Can you work these out from the model? Positions are in its coordinate system, mm. Face numbers are marked on the shaded views. Give positions to 0.01 mm unless a question says otherwise; leave off trailing zeros. Loops run counter-clockwise (first coordinate to the right, second up) from the corner with the lowest first, then second, coordinate; pieces in that order, holes last. Notation, with made-up numbers: (87.25, 30.5) -> (118.25, 30.5) arc R28 ccw to (118.25, 62.5) -> close; hole circle Ø10 at (35, 21.25). An arc over 180 degrees is marked (long way). One line per question, with ' | ' between items.
from build123d import *

# Parameters (mm, degrees)
SKETCH1_W                     = 22.225
SKETCH1_H                     = 15.875
SKETCH1_R                     = 1.5875
BOSS_EXTRUDE1_DEPTH           = 1
SKETCH2_W                     = 3
SKETCH2_H                     = 4
BOSS_EXTRUDE2_DEPTH           = 1
SKETCH3_R                     = 1.27
BOSS_EXTRUDE3_DEPTH           = 1
BOSS_EXTRUDE3_DRAFT           = 40
BOSS_EXTRUDE3_PROFILE_2_DEPTH = 1
BOSS_EXTRUDE3_PROFILE_2_DRAFT = 40
BOSS_EXTRUDE3_PROFILE_3_DEPTH = 1
BOSS_EXTRUDE3_PROFILE_3_DRAFT = 40
BOSS_EXTRUDE3_PROFILE_4_DEPTH = 1
BOSS_EXTRUDE3_PROFILE_4_DRAFT = 40
BOSS_EXTRUDE3_PROFILE_5_DEPTH = 1
BOSS_EXTRUDE3_PROFILE_5_DRAFT = 40
BOSS_EXTRUDE3_PROFILE_6_DEPTH = 1
BOSS_EXTRUDE3_PROFILE_6_DRAFT = 40
BOSS_EXTRUDE3_PROFILE_7_DEPTH = 1
BOSS_EXTRUDE3_PROFILE_7_DRAFT = 40
BOSS_EXTRUDE3_PROFILE_8_DEPTH = 1
BOSS_EXTRUDE3_PROFILE_8_DRAFT = 40
SKETCH4_R                     = 0.430900369
BOSS_EXTRUDE4_DEPTH           = 9.89


with BuildPart() as part:
    # Sketch1 → Boss-Extrude1 (new body)
    with BuildSketch(Plane.XY):
        with Locations((-11.1125, 7.9375)):
            Rectangle(SKETCH1_W, SKETCH1_H)
        with Locations((-18.7325, 3.4925)):
            Circle(SKETCH1_R, mode=Mode.SUBTRACT)
        with Locations((-3.4925, 3.4925)):
            Circle(SKETCH1_R, mode=Mode.SUBTRACT)
    extrude(amount=BOSS_EXTRUDE1_DEPTH)

    # Sketch2 → Boss-Extrude2 (add)
    with BuildSketch(Plane.XY):
        with Locations((-11.1125, 9.812715541)):
            Rectangle(SKETCH2_W, SKETCH2_H)
    extrude(amount=-BOSS_EXTRUDE2_DEPTH)


with BuildPart() as boss_extrude3_tool:
    # Sketch3 → Boss-Extrude3 (with draft: the straight prism first)
    with BuildSketch(Plane.XY.offset(1)):
        with Locations((-20.955, 14.605)):
            Circle(SKETCH3_R)
    extrude(amount=BOSS_EXTRUDE3_DEPTH)
    # Boss-Extrude3: the draft: its side faces are tilted about the plane it starts from
    boss_extrude3_sides = [boss_extrude3_tool.faces().sort_by_distance(p)[0] for p in [
        (-22.225, 14.605, 1.5),
    ]]
    draft(boss_extrude3_sides, Plane.XY.offset(1), BOSS_EXTRUDE3_DRAFT)


with BuildPart() as part_1:
    add(part.part)

    # Boss-Extrude3: add boss_extrude3_tool
    add(boss_extrude3_tool.part)


with BuildPart() as boss_extrude3_profile_2_tool:
    # Sketch3 → Boss-Extrude3 profile 2 (with draft: the straight prism first)
    with BuildSketch(Plane.XY.offset(1)):
        with Locations((-18.142857143, 14.605)):
            Circle(SKETCH3_R)
    extrude(amount=BOSS_EXTRUDE3_PROFILE_2_DEPTH)
    # Boss-Extrude3 profile 2: the draft: its side faces are tilted about the plane it starts from
    boss_extrude3_profile_2_sides = [boss_extrude3_profile_2_tool.faces().sort_by_distance(p)[0] for p in [
        (-19.412857143, 14.605, 1.5),
    ]]
    draft(boss_extrude3_profile_2_sides, Plane.XY.offset(1), BOSS_EXTRUDE3_PROFILE_2_DRAFT)


with BuildPart() as part_2:
    add(part_1.part)

    # Boss-Extrude3 profile 2: add boss_extrude3_profile_2_tool
    add(boss_extrude3_profile_2_tool.part)


with BuildPart() as boss_extrude3_profile_3_tool:
    # Sketch3 → Boss-Extrude3 profile 3 (with draft: the straight prism first)
    with BuildSketch(Plane.XY.offset(1)):
        with Locations((-15.330714286, 14.605)):
            Circle(SKETCH3_R)
    extrude(amount=BOSS_EXTRUDE3_PROFILE_3_DEPTH)
    # Boss-Extrude3 profile 3: the draft: its side faces are tilted about the plane it starts from
    boss_extrude3_profile_3_sides = [boss_extrude3_profile_3_tool.faces().sort_by_distance(p)[0] for p in [
        (-16.600714286, 14.605, 1.5),
    ]]
    draft(boss_extrude3_profile_3_sides, Plane.XY.offset(1), BOSS_EXTRUDE3_PROFILE_3_DRAFT)


with BuildPart() as part_3:
    add(part_2.part)

    # Boss-Extrude3 profile 3: add boss_extrude3_profile_3_tool
    add(boss_extrude3_profile_3_tool.part)


with BuildPart() as boss_extrude3_profile_4_tool:
    # Sketch3 → Boss-Extrude3 profile 4 (with draft: the straight prism first)
    with BuildSketch(Plane.XY.offset(1)):
        with Locations((-12.518571429, 14.605)):
            Circle(SKETCH3_R)
    extrude(amount=BOSS_EXTRUDE3_PROFILE_4_DEPTH)
    # Boss-Extrude3 profile 4: the draft: its side faces are tilted about the plane it starts from
    boss_extrude3_profile_4_sides = [boss_extrude3_profile_4_tool.faces().sort_by_distance(p)[0] for p in [
        (-13.788571429, 14.605, 1.5),
    ]]
    draft(boss_extrude3_profile_4_sides, Plane.XY.offset(1), BOSS_EXTRUDE3_PROFILE_4_DRAFT)


with BuildPart() as part_4:
    add(part_3.part)

    # Boss-Extrude3 profile 4: add boss_extrude3_profile_4_tool
    add(boss_extrude3_profile_4_tool.part)


with BuildPart() as boss_extrude3_profile_5_tool:
    # Sketch3 → Boss-Extrude3 profile 5 (with draft: the straight prism first)
    with BuildSketch(Plane.XY.offset(1)):
        with Locations((-9.706428571, 14.605)):
            Circle(SKETCH3_R)
    extrude(amount=BOSS_EXTRUDE3_PROFILE_5_DEPTH)
    # Boss-Extrude3 profile 5: the draft: its side faces are tilted about the plane it starts from
    boss_extrude3_profile_5_sides = [boss_extrude3_profile_5_tool.faces().sort_by_distance(p)[0] for p in [
        (-10.976428571, 14.605, 1.5),
    ]]
    draft(boss_extrude3_profile_5_sides, Plane.XY.offset(1), BOSS_EXTRUDE3_PROFILE_5_DRAFT)


with BuildPart() as part_5:
    add(part_4.part)

    # Boss-Extrude3 profile 5: add boss_extrude3_profile_5_tool
    add(boss_extrude3_profile_5_tool.part)


with BuildPart() as boss_extrude3_profile_6_tool:
    # Sketch3 → Boss-Extrude3 profile 6 (with draft: the straight prism first)
    with BuildSketch(Plane.XY.offset(1)):
        with Locations((-6.894285714, 14.605)):
            Circle(SKETCH3_R)
    extrude(amount=BOSS_EXTRUDE3_PROFILE_6_DEPTH)
    # Boss-Extrude3 profile 6: the draft: its side faces are tilted about the plane it starts from
    boss_extrude3_profile_6_sides = [boss_extrude3_profile_6_tool.faces().sort_by_distance(p)[0] for p in [
        (-8.164285714, 14.605, 1.5),
    ]]
    draft(boss_extrude3_profile_6_sides, Plane.XY.offset(1), BOSS_EXTRUDE3_PROFILE_6_DRAFT)


with BuildPart() as part_6:
    add(part_5.part)

    # Boss-Extrude3 profile 6: add boss_extrude3_profile_6_tool
    add(boss_extrude3_profile_6_tool.part)


with BuildPart() as boss_extrude3_profile_7_tool:
    # Sketch3 → Boss-Extrude3 profile 7 (with draft: the straight prism first)
    with BuildSketch(Plane.XY.offset(1)):
        with Locations((-4.082142857, 14.605)):
            Circle(SKETCH3_R)
    extrude(amount=BOSS_EXTRUDE3_PROFILE_7_DEPTH)
    # Boss-Extrude3 profile 7: the draft: its side faces are tilted about the plane it starts from
    boss_extrude3_profile_7_sides = [boss_extrude3_profile_7_tool.faces().sort_by_distance(p)[0] for p in [
        (-5.352142857, 14.605, 1.5),
    ]]
    draft(boss_extrude3_profile_7_sides, Plane.XY.offset(1), BOSS_EXTRUDE3_PROFILE_7_DRAFT)


with BuildPart() as part_7:
    add(part_6.part)

    # Boss-Extrude3 profile 7: add boss_extrude3_profile_7_tool
    add(boss_extrude3_profile_7_tool.part)


with BuildPart() as boss_extrude3_profile_8_tool:
    # Sketch3 → Boss-Extrude3 profile 8 (with draft: the straight prism first)
    with BuildSketch(Plane.XY.offset(1)):
        with Locations((-1.27, 14.605)):
            Circle(SKETCH3_R)
    extrude(amount=BOSS_EXTRUDE3_PROFILE_8_DEPTH)
    # Boss-Extrude3 profile 8: the draft: its side faces are tilted about the plane it starts from
    boss_extrude3_profile_8_sides = [boss_extrude3_profile_8_tool.faces().sort_by_distance(p)[0] for p in [
        (-2.54, 14.605, 1.5),
    ]]
    draft(boss_extrude3_profile_8_sides, Plane.XY.offset(1), BOSS_EXTRUDE3_PROFILE_8_DRAFT)


with BuildPart() as part_8:
    add(part_7.part)

    # Boss-Extrude3 profile 8: add boss_extrude3_profile_8_tool
    add(boss_extrude3_profile_8_tool.part)

    # Sketch4 → Boss-Extrude4 (add)
    with BuildSketch(Plane.XY.offset(2)):
        with Locations((-20.955, 14.605)):
            Circle(SKETCH4_R)
        with Locations((-18.142857143, 14.605)):
            Circle(SKETCH4_R)
        with Locations((-15.330714286, 14.605)):
            Circle(SKETCH4_R)
        with Locations((-12.518571429, 14.605)):
            Circle(SKETCH4_R)
        with Locations((-9.706428571, 14.605)):
            Circle(SKETCH4_R)
        with Locations((-6.894285714, 14.605)):
            Circle(SKETCH4_R)
        with Locations((-4.082142857, 14.605)):
            Circle(SKETCH4_R)
        with Locations((-1.27, 14.605)):
            Circle(SKETCH4_R)
    extrude(amount=-BOSS_EXTRUDE4_DEPTH)


solid = part_8.part
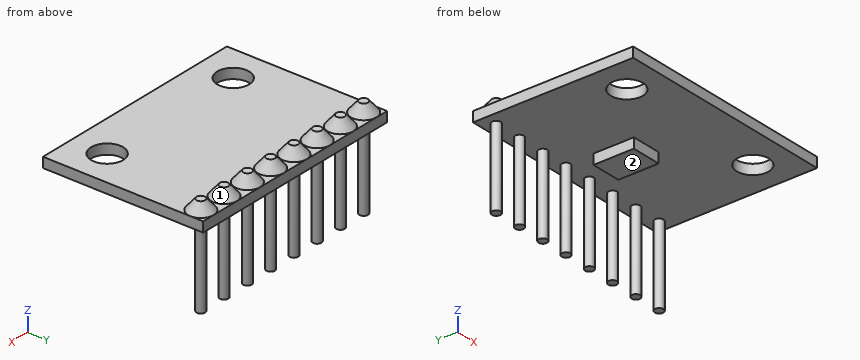
Q1. If I drill on probe 1 along Z at (x, y) = (-7, 5.5); probe 2 along X at (y, z) = (11.75, -0.5); probe 3 along Y at (x, z) = (-20.75, -4), over which ranges is the centre line in solid material (lowest first)? Write a range as from..to.
Entries:
probe 1: 0..1 | probe 2: -12.61..-9.61 | probe 3: 14.23..14.98
Q2. For pin 1 Ø0.8 at (x, z) = (-10.5, -0.5) entering from -Y; pin 2 Ø0.8 at (y, z) = (9, -0.5) entering from -X; pin 3 Ø4 at (x, y) = (-7, 12) entering from -Z; pin 4 Ø2 at (x, y) = (-10, 14) entering from +Z, each with a flat end and sliding along its axis, tell me the tip position at first contact or that it passes through.
Entries:
pin 1: y = 7.81 | pin 2: x = -12.61 | pin 3: z = 0 | pin 4: z = 2
Q3. If we section it at C-C (y = 4.5): Write out the boundary of the cut face in (x, z) (3 decimals).
Entries:
outline: (-22.225, 0) -> (-19.959, 0) -> (-19.959, 1) -> (-22.225, 1) -> close; (-17.506, 0) -> (-4.719, 0) -> (-4.719, 1) -> (-17.506, 1) -> close; (-2.266, 0) -> (0, 0) -> (0, 1) -> (-2.266, 1) -> close
Q4. If we mould it in two halves opening along X, with no side actions, what happens to the marked faces 1 and 2? For each: pulls with the +X half, pulls with the -X half, needs draft (parallel to the pull), parting line crosses it, or undercut.
Entries:
face 1: undercut | face 2: needs draft
Q5. If we section it at A-A (z = -4.25): Write out the boundary of the cut face in (x, y) (3 decimals).
Entries:
outline: circle Ø0.862 at (-20.955, 14.605); circle Ø0.862 at (-18.143, 14.605); circle Ø0.862 at (-15.331, 14.605); circle Ø0.862 at (-12.519, 14.605); circle Ø0.862 at (-9.706, 14.605); circle Ø0.862 at (-6.894, 14.605); circle Ø0.862 at (-4.082, 14.605); circle Ø0.862 at (-1.27, 14.605)
Q6. If we section it at D-D (z = 0.75): Write out the boundary of the cut face in (x, y) (1 decimal), plus the area to 3 significant figures.
Entries:
outline: (-22.2, 0) -> (0, 0) -> (0, 15.9) -> (-22.2, 15.9) -> close; hole circle Ø3.2 at (-18.7, 3.5); hole circle Ø3.2 at (-3.5, 3.5) | area: 337 mm²
Q7. If we section it at B-B (y = 10): Write out the boundary of the cut face in (x, z) (1 decimal).
Entries:
outline: (-22.2, 0) -> (-12.6, 0) -> (-12.6, -1) -> (-9.6, -1) -> (-9.6, 0) -> (0, 0) -> (0, 1) -> (-22.2, 1) -> close
